Part model, mm, in its own coordinate system. Face numbers are marked on the shaded views. A direction names the side the tool comes from. Give positions to 0.01 mm unless a question says otherwise; leave off trailing zeros. Order: outer loops, then holes, each group sorted by start corner. A loop starts at its lowest first (then second) coordinate and runs counter-clockwise, first axis right, second up. Notation, with made-up numbers: (12.25, 31) - (26.25, 31) arc R7 cw to (26.25, 40) - close; hole circle Ø10 at (-10.75, 21.5). An arc over 180 degrees is marked (long way). Use one line per item in the form item = value. Start each with the question number.
1. Band-saw the part on C-C, the plane x = -1. List the corners of the cut face in (y, z), plus the area to 3 significant figures.
2. Band-saw the part on B-B, the plane x = 7. List the corners of the cut face in (y, z), plus the area to 3 significant figures.
3. Pin check, flat tips, straight feed: P1, Ø4.5, axis at y = 3.19, z = 47.13, coming from the +X side; P2, Ø1.3, axis at y = 4, z = 32, coming from the +X side; P3, Ø5, axis at x = 7.5, z = 32.5, coming from the -Y side; P4, Ø4, axis at x = -1, y = 2.5, coming from the -Z side. Stop position of each tip, or through.
4. Tool access for the marked faces 4 and 5: list every direction of +Z, -Z, +X, -X, +Y, -Y with a clear straight run to the whole face (end or side of a thin tool).
5. Pull direction Y, two halves, no side cores. Call the marked faces 1, 2 and 3: +Y half, -Y half, draft (parallel to the pull), parting line (faces both ways), or undercut.
6. Band-saw the part on D-D, the plane y = 13.5. List the corners of the cut face in (x, z).
7. Band-saw the part on A-A, the plane z = 34. List the corners of the cut face in (x, y), plus the area to 3 significant figures.
8. Drill centre lines: line 1 (Y direction, x = 4, z = 35); line 2 (Y direction, x = 2.5, z = 32.5); line 3 (Z direction, x = 2.75, y = 10). Where is each one in solid material? Low to high.
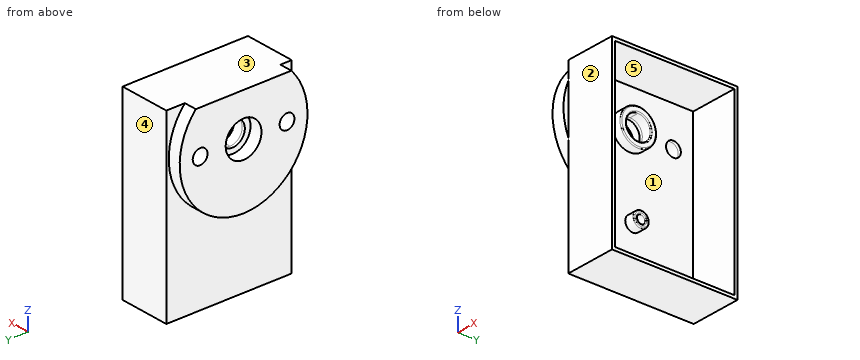
Autodesk Inventor part; units mm, degrees
ref_plane "YZ Plane" through (0, 0, 0) normal (1, 0, 0) x (0, 1, 0)
ref_plane "XZ Plane" through (0, 0, 0) normal (0, 1, 0) x (-1, 0, 0)
ref_plane "XY Plane" through (0, 0, 0) normal (0, 0, 1) x (1, 0, 0)
sketch "Sketch1" plane through (0, 0, 0) normal (1, 0, 0) x (0, 1, 0)
  circle A0 centre (3.7472, 31.8344) radius 0.7
  arc A1 (6.295, 21.1336) -> (6.4355, 23.5076) centre (-1.824, 22.8051) ccw
  arc A2 (5.4476, 20.9667) -> (6.295, 21.1336) centre (3.7472, 31.8344) ccw
  arc A3 (4.4173, 23.1101) -> (5.4476, 20.9667) centre (12.3263, 25.5922) ccw
  arc A4 (3.7308, 23.0845) -> (4.4173, 23.1101) centre (3.7472, 31.8344) ccw
  arc A5 (2.8636, 20.87) -> (3.7308, 23.0845) centre (-4.3415, 24.9686) ccw
  arc A6 (2.006, 20.9731) -> (2.8636, 20.87) centre (3.7472, 31.8344) ccw
  arc A7 (1.6886, 23.33) -> (2.006, 20.9731) centre (9.9774, 23.2466) ccw
  arc A8 (1.0277, 23.5178) -> (1.6886, 23.33) centre (3.7472, 31.8344) ccw
  arc A9 (-0.4814, 21.6797) -> (1.0277, 23.5178) centre (-6.0673, 27.8042) ccw
  arc A10 (-1.2651, 22.0427) -> (-0.4814, 21.6797) centre (3.7472, 31.8344) ccw
  arc A11 (-0.8387, 24.3824) -> (-1.2651, 22.0427) centre (7.0187, 21.7417) ccw
  arc A12 (-1.4092, 24.7652) -> (-0.8387, 24.3824) centre (3.7472, 31.8344) ccw
  arc A13 (-3.4124, 23.4834) -> (-1.4092, 24.7652) centre (-6.8324, 31.0342) ccw
  arc A14 (-4.0456, 24.0709) -> (-3.4124, 23.4834) centre (3.7472, 31.8344) ccw
  arc A15 (-2.917, 26.1642) -> (-4.0456, 24.0709) centre (3.7397, 21.2247) ccw
  arc A16 (-3.3414, 26.7046) -> (-2.917, 26.1642) centre (3.7472, 31.8344) ccw
  arc A17 (-5.6426, 26.1045) -> (-3.3414, 26.7046) centre (-6.5618, 34.3427) ccw
  arc A18 (-6.0632, 26.8589) -> (-5.6426, 26.1045) centre (3.7472, 31.8344) ccw
  arc A19 (-4.343, 28.5011) -> (-6.0632, 26.8589) centre (0.4615, 21.7463) ccw
  arc A20 (-4.5796, 29.1461) -> (-4.343, 28.5011) centre (3.7472, 31.8344) ccw
  arc A21 (-6.9537, 29.2866) -> (-4.5796, 29.1461) centre (-5.2822, 37.4056) ccw
  arc A22 (-7.1206, 30.134) -> (-6.9537, 29.2866) centre (3.7472, 31.8344) ccw
  arc A23 (-4.9771, 31.1643) -> (-7.1206, 30.134) centre (-2.4951, 23.2553) ccw
  arc A24 (-5.0028, 31.8508) -> (-4.9771, 31.1643) centre (3.7472, 31.8344) ccw
  arc A25 (-7.2173, 32.718) -> (-5.0028, 31.8508) centre (-3.1187, 39.9231) ccw
  arc A26 (-7.1142, 33.5756) -> (-7.2173, 32.718) centre (3.7472, 31.8344) ccw
  arc A27 (-4.7572, 33.893) -> (-7.1142, 33.5756) centre (-4.8407, 25.6042) ccw
  arc A28 (-4.5695, 34.5539) -> (-4.7572, 33.893) centre (3.7472, 31.8344) ccw
  arc A29 (-6.4076, 36.063) -> (-4.5695, 34.5539) centre (-0.2831, 41.6489) ccw
  arc A30 (-6.0445, 36.8467) -> (-6.4076, 36.063) centre (3.7472, 31.8344) ccw
  arc A31 (-3.7048, 36.4203) -> (-6.0445, 36.8467) centre (-6.3456, 28.5629) ccw
  arc A32 (-3.3221, 36.9908) -> (-3.7048, 36.4203) centre (3.7472, 31.8344) ccw
  arc A33 (-4.6039, 38.994) -> (-3.3221, 36.9908) centre (2.947, 42.414) ccw
  arc A34 (-4.0164, 39.6272) -> (-4.6039, 38.994) centre (3.7472, 31.8344) ccw
  arc A35 (-1.923, 38.4986) -> (-4.0164, 39.6272) centre (-6.8626, 31.8419) ccw
  arc A36 (-1.3827, 38.923) -> (-1.923, 38.4986) centre (3.7472, 31.8344) ccw
  arc A37 (-1.9827, 41.2242) -> (-1.3827, 38.923) centre (6.2554, 42.1434) ccw
  arc A38 (-1.2283, 41.6448) -> (-1.9827, 41.2242) centre (3.7472, 31.8344) ccw
  arc A39 (0.4139, 39.9246) -> (-1.2283, 41.6448) centre (-6.341, 35.1201) ccw
  arc A40 (1.0589, 40.1612) -> (0.4139, 39.9246) centre (3.7472, 31.8344) ccw
  arc A41 (1.1993, 42.5353) -> (1.0589, 40.1612) centre (9.3183, 40.8638) ccw
  arc A42 (2.0468, 42.7022) -> (1.1993, 42.5353) centre (3.7472, 31.8344) ccw
  arc A43 (3.077, 40.5587) -> (2.0468, 42.7022) centre (-4.8319, 38.0767) ccw
  arc A44 (3.7636, 40.5844) -> (3.077, 40.5587) centre (3.7472, 31.8344) ccw
  arc A45 (4.6308, 42.7989) -> (3.7636, 40.5844) centre (11.8359, 38.7003) ccw
  arc A46 (5.4883, 42.6958) -> (4.6308, 42.7989) centre (3.7472, 31.8344) ccw
  arc A47 (5.8058, 40.3388) -> (5.4883, 42.6958) centre (-2.4831, 40.4223) ccw
  arc A48 (6.4667, 40.1511) -> (5.8058, 40.3388) centre (3.7472, 31.8344) ccw
  arc A49 (7.9757, 41.9892) -> (6.4667, 40.1511) centre (13.5616, 35.8647) ccw
  arc A50 (8.7594, 41.6261) -> (7.9757, 41.9892) centre (3.7472, 31.8344) ccw
  arc A51 (8.333, 39.2865) -> (8.7594, 41.6261) centre (0.4756, 41.9272) ccw
  arc A52 (8.9036, 38.9037) -> (8.333, 39.2865) centre (3.7472, 31.8344) ccw
  arc A53 (10.9068, 40.1855) -> (8.9036, 38.9037) centre (14.3267, 32.6346) ccw
  arc A54 (11.5399, 39.598) -> (10.9068, 40.1855) centre (3.7472, 31.8344) ccw
  arc A55 (10.4114, 37.5046) -> (11.5399, 39.598) centre (3.7546, 42.4442) ccw
  arc A56 (10.8357, 36.9643) -> (10.4114, 37.5046) centre (3.7472, 31.8344) ccw
  arc A57 (13.137, 37.5643) -> (10.8357, 36.9643) centre (14.0562, 29.3262) ccw
  arc A58 (13.5576, 36.81) -> (13.137, 37.5643) centre (3.7472, 31.8344) ccw
  arc A59 (11.8374, 35.1678) -> (13.5576, 36.81) centre (7.0328, 41.9226) ccw
  arc A60 (12.074, 34.5227) -> (11.8374, 35.1678) centre (3.7472, 31.8344) ccw
  arc A61 (14.448, 34.3823) -> (12.074, 34.5227) centre (12.7765, 26.2633) ccw
  arc A62 (14.615, 33.5348) -> (14.448, 34.3823) centre (3.7472, 31.8344) ccw
  arc A63 (12.4715, 32.5046) -> (14.615, 33.5348) centre (9.9894, 40.4135) ccw
  arc A64 (12.4972, 31.818) -> (12.4715, 32.5046) centre (3.7472, 31.8344) ccw
  arc A65 (14.7116, 30.9508) -> (12.4972, 31.818) centre (10.613, 23.7458) ccw
  arc A66 (14.6085, 30.0933) -> (14.7116, 30.9508) centre (3.7472, 31.8344) ccw
  arc A67 (12.2516, 29.7758) -> (14.6085, 30.0933) centre (12.335, 38.0647) ccw
  arc A68 (12.0638, 29.1149) -> (12.2516, 29.7758) centre (3.7472, 31.8344) ccw
  arc A69 (13.9019, 27.6059) -> (12.0638, 29.1149) centre (7.7775, 22.02) ccw
  arc A70 (13.5389, 26.8222) -> (13.9019, 27.6059) centre (3.7472, 31.8344) ccw
  arc A71 (11.1992, 27.2486) -> (13.5389, 26.8222) centre (13.8399, 35.106) ccw
  arc A72 (10.8164, 26.6781) -> (11.1992, 27.2486) centre (3.7472, 31.8344) ccw
  arc A73 (12.0982, 24.6748) -> (10.8164, 26.6781) centre (4.5474, 21.2549) ccw
  arc A74 (11.5108, 24.0417) -> (12.0982, 24.6748) centre (3.7472, 31.8344) ccw
  arc A75 (9.4174, 25.1702) -> (11.5108, 24.0417) centre (14.3569, 31.827) ccw
  arc A76 (8.877, 24.7459) -> (9.4174, 25.1702) centre (3.7472, 31.8344) ccw
  arc A77 (9.4771, 22.4446) -> (8.877, 24.7459) centre (1.2389, 21.5254) ccw
  arc A78 (8.7227, 22.024) -> (9.4771, 22.4446) centre (3.7472, 31.8344) ccw
  arc A79 (7.0805, 23.7442) -> (8.7227, 22.024) centre (13.8353, 28.5488) ccw
  arc A80 (6.4355, 23.5076) -> (7.0805, 23.7442) centre (3.7472, 31.8344) ccw
  line L0 (4.9954, 45.8746) -> (4.8965, 48.5188)
  arc A81 (4.8965, 48.5188) -> (4.9954, 45.8746) centre (3.1894, 47.131) ccw
  arc A82 (-0.8751, 51.5446) -> (0.2488, 49.4581) centre (4.3942, 53.0372) ccw
  arc A83 (-0.1346, 52.1261) -> (-0.8751, 51.5446) centre (3.1894, 47.131) ccw
  arc A84 (1.6258, 50.5395) -> (-0.1346, 52.1261) centre (-2.834, 47.3609) ccw
  arc A85 (2.1783, 50.7421) -> (1.6258, 50.5395) centre (3.1894, 47.131) ccw
  arc A86 (2.4954, 53.0907) -> (2.1783, 50.7421) centre (7.6357, 51.201) ccw
  arc A87 (3.4362, 53.1259) -> (2.4954, 53.0907) centre (3.1894, 47.131) ccw
  arc A88 (3.9279, 50.8076) -> (3.4362, 53.1259) centre (-1.5485, 50.8574) ccw
  arc A89 (4.4939, 50.6468) -> (3.9279, 50.8076) centre (3.1894, 47.131) ccw
  arc A90 (6.131, 52.3605) -> (4.4939, 50.6468) centre (9.1788, 47.8103) ccw
  arc A91 (6.9128, 51.8359) -> (6.131, 52.3605) centre (3.1894, 47.131) ccw
  arc A92 (5.9479, 49.6713) -> (6.9128, 51.8359) centre (1.5467, 52.9306) ccw
  arc A93 (6.3113, 49.2085) -> (5.9479, 49.6713) centre (3.1894, 47.131) ccw
  arc A94 (8.643, 49.6327) -> (6.3113, 49.2085) centre (8.4342, 44.1601) ccw
  arc A95 (8.9672, 48.7488) -> (8.643, 49.6327) centre (3.1894, 47.131) ccw
  arc A96 (6.9142, 47.5648) -> (8.9672, 48.7488) centre (5.2694, 52.7886) ccw
  arc A97 (6.9362, 46.9768) -> (6.9142, 47.5648) centre (3.1894, 47.131) ccw
  arc A98 (9.0719, 45.9494) -> (6.9362, 46.9768) centre (5.6863, 41.6447) ccw
  arc A99 (8.8147, 45.0438) -> (9.0719, 45.9494) centre (3.1894, 47.131) ccw
  arc A100 (6.4578, 45.2925) -> (8.8147, 45.0438) centre (8.1976, 50.4855) ccw
  arc A101 (6.13, 44.8039) -> (6.4578, 45.2925) centre (3.1894, 47.131) ccw
  arc A102 (7.254, 42.7174) -> (6.13, 44.8039) centre (1.9846, 41.2248) ccw
  arc A103 (6.5135, 42.1359) -> (7.254, 42.7174) centre (3.1894, 47.131) ccw
  arc A104 (4.753, 43.7225) -> (6.5135, 42.1359) centre (9.2128, 46.9012) ccw
  arc A105 (4.2006, 43.5199) -> (4.753, 43.7225) centre (3.1894, 47.131) ccw
  arc A106 (3.8835, 41.1713) -> (4.2006, 43.5199) centre (-1.2568, 43.061) ccw
  arc A107 (2.9426, 41.1361) -> (3.8835, 41.1713) centre (3.1894, 47.131) ccw
  arc A108 (2.4509, 43.4544) -> (2.9426, 41.1361) centre (7.9274, 43.4046) ccw
  arc A109 (1.8849, 43.6152) -> (2.4509, 43.4544) centre (3.1894, 47.131) ccw
  arc A110 (0.2479, 41.9015) -> (1.8849, 43.6152) centre (-2.8, 46.4517) ccw
  arc A111 (-0.534, 42.4261) -> (0.2479, 41.9015) centre (3.1894, 47.131) ccw
  arc A112 (0.4309, 44.5907) -> (-0.534, 42.4261) centre (4.8322, 41.3314) ccw
  arc A113 (0.0675, 45.0535) -> (0.4309, 44.5907) centre (3.1894, 47.131) ccw
  arc A114 (-2.2641, 44.6293) -> (0.0675, 45.0535) centre (-2.0554, 50.1019) ccw
  arc A115 (-2.5884, 45.5132) -> (-2.2641, 44.6293) centre (3.1894, 47.131) ccw
  arc A116 (-0.5354, 46.6972) -> (-2.5884, 45.5132) centre (1.1095, 41.4734) ccw
  arc A117 (-0.5574, 47.2852) -> (-0.5354, 46.6972) centre (3.1894, 47.131) ccw
  arc A118 (-2.6931, 48.3126) -> (-0.5574, 47.2852) centre (0.6926, 52.6173) ccw
  arc A119 (-2.4358, 49.2183) -> (-2.6931, 48.3126) centre (3.1894, 47.131) ccw
  arc A120 (-0.079, 48.9695) -> (-2.4358, 49.2183) centre (-1.8187, 43.7765) ccw
  arc A121 (0.2488, 49.4581) -> (-0.079, 48.9695) centre (3.1894, 47.131) ccw
  line L1 (16.152, 19.5075) -> (-8.3796, 19.5075)
  line L2 (-8.3796, 19.5075) -> (-8.3796, 55.4678)
  line L3 (-8.3796, 55.4678) -> (16.152, 55.4678)
  line L4 (16.152, 55.4678) -> (16.152, 19.5075)
  point P0 (0, 0)
extrude "Extrusion1" add sketch "Sketch1" along normal blind 10 contours A0 | A2 A3 A4 A5 A6 A7 A8 A9 A10 A11 A12 A13 A14 A15 A16 A17 A18 A19 A20 A21 A22 A23 A24 A25 A26 A27 A28 A29 A30 A31 A32 A33 A34 A35 A36 A37 A38 A39 A40 A41 A42 A43 A44 A45 A46 A47 A48 A49 A50 A51 A52 A53 A54 A55 A56 A57 A58 A59 A60 A61 A62 A63 A64 A65 A66 A67 A68 A69 A70 A71 A72 A73 A74 A75 A76 A77 A78 A79 A80 A1 | A81 L0 | A83 A84 A85 A86 A87 A88 A89 A90 A91 A92 A93 A94 A95 A96 A97 A98 A99 A100 A101 A102 A103 A104 A105 A106 A107 A108 A109 A110 A111 A112 A113 A114 A115 A116 A117 A118 A119 A120 A121 A82 | L1 L2 L3 L4
shell "Shell1" thickness 0.6 removed faces 1 at (10, -0.2024, 43.481)
sketch "Sketch3" plane through (0.6, -7.7796, 20.1075) normal (1, 0, 0) x (0, 0, -1)
  circle A0 centre (-11.7269, 11.5268) radius 0.8
  circle A1 centre (-27.0563, 10.9578) radius 3.5
  circle A2 centre (-11.7269, 11.5268) radius 1.5
  circle A3 centre (-27.0235, 10.969) radius 2.4
  point P0 (20.1075, 7.7796)
  dimension "d3" = 3
  dimension "d19" = 4.8
  dimension "d20" = 1.6
extrude "Extrusion3" add sketch "Sketch3" along normal blind 2
fillet "Fillet1" radius 0.2 4 edges at (2.6, 3.1894, 49.531) (2.6, 3.1782, 50.6638) (2.6, 3.7472, 32.6344) (2.6, 3.7472, 33.3344)
sketch "Sketch4" plane through (0, 0, 0) normal (-1, 0, 0) x (0, 0, 1)
  circle A0 centre (47.1638, -5.3218) radius 1.45
  circle A1 centre (47.1638, 11.6782) radius 1.45
  point P0 (0, 0)
  dimension "d13" = 2.9
  dimension "d14" = 2.9
extrude "Extrusion4" cut sketch "Sketch4" against normal through all
sketch "Sketch5" plane through (0, 0, 0) normal (-1, 0, 0) x (0, 0, 1)
  circle A0 centre (47.1638, 3.1782) radius 3.5
  circle A1 centre (47.1638, 3.1782) radius 12.5
  circle A2 centre (47.1638, 11.6782) radius 1.45
  circle A3 centre (47.1638, -5.3218) radius 1.25
  line L0 (55.4678, -8.3796) -> (55.4678, 16.152)
  line L1 (55.4678, -6.1649) -> (55.4678, 12.5213)
  point P0 (0, 0)
extrude "Extrusion5" add sketch "Sketch5" along normal blind 2.5 contours L0 A1 picked at (53.8665, 3.1782)
sketch "Sketch7" plane through (-2.5, 0, 0) normal (-1, 0, 0) x (0, 0, 1)
  circle A0 centre (47.1638, 3.1782) radius 3.5
  circle A1 centre (47.131, 3.1894) radius 2.4
  point P0 (0, 0)
extrude "Extrusion7" cut sketch "Sketch7" against normal through all contours A1
sketch "Sketch8" plane through (-2.5, 0, 0) normal (-1, 0, 0) x (0, 0, 1)
  circle A0 centre (47.1638, -5.3218) radius 1.45
  point P0 (0, 0)
extrude "Extrusion8" cut sketch "Sketch8" against normal through all
properties part number "GearHolder"
From the geometry:
q1.outline = (-6.16, 55.47) arc R12.5 ccw (long way) to (12.52, 55.47) - close; hole circle Ø2.9 at (-5.32, 47.16); hole circle Ø7 at (3.18, 47.16); hole circle Ø2.9 at (11.68, 47.16)
q1.area = 385 mm²
q2.outline = (-8.38, 19.51) - (16.15, 19.51) - (16.15, 55.47) - (-8.38, 55.47) - close; hole (-7.78, 20.11) - (15.55, 20.11) - (15.55, 54.87) - (-7.78, 54.87) - close
q2.area = 71.2 mm²
q3.P1 = through
q3.P2 = 2.59
q3.P3 = -8.38
q3.P4 = 19.51
q4.face_4 = +Z, -Z, +X, -X, +Y
q4.face_5 = +X
q5.face_1 = undercut
q5.face_2 = -Y half
q5.face_3 = draft
q6.outline = (-2.5, 40.11) - (0, 40.11) - (0, 19.51) - (10, 19.51) - (10, 20.11) - (0.6, 20.11) - (0.6, 54.87) - (10, 54.87) - (10, 55.47) - (0, 55.47) - (0, 54.21) - (-2.5, 54.21) - close
q7.outline = (0, -8.38) - (10, -8.38) - (10, -7.78) - (0.6, -7.78) - (0.6, 15.55) - (10, 15.55) - (10, 16.15) - (0, 16.15) - close
q7.area = 26.0 mm²
q8.line_1 = -8.38 to -7.78, 15.55 to 16.15
q8.line_2 = -8.38 to -7.78, 2.43 to 3.26, 4.24 to 5.06, 15.55 to 16.15
q8.line_3 = 19.51 to 20.11, 54.87 to 55.47
